from build123d import *

# Parameters (mm, degrees)
F1_DEPTH  = 1000
F2_T      = -3
F3_W      = 300
F3_H      = 3
F4_DEPTH  = 300
F6_DEPTH  = 5
F8_DEPTH  = 5
F9_W      = 100
F9_H      = 1500
F10_DEPTH = 100
F12_DEPTH = 800.001
F13_W     = 100
F13_H     = 1500
F14_DEPTH = 100
F16_DEPTH = 1100.001
F17_W     = 290
F17_H     = 3
F18_DEPTH = 300
F20_DEPTH = 5
F22_DEPTH = 5
F24_DEPTH = 100
F26_DEPTH = 100
F28_DEPTH = 744.22
F29_W     = 284.3456985965
F29_H     = 700
F30_DEPTH = 25.4


with BuildPart() as f1:
    # F0 (on Right) → F1 (new body)
    with BuildSketch(Plane.YZ):
        with BuildLine():
            Line((250, 100), (250, 600))
            Line((250, 600), (-250, 600))
            Line((-250, 600), (-250, 100))
            ThreePointArc((-250, 100), (-220.7106781187, 29.2893218813), (-150, 0))
            Line((-150, 0), (150, 0))
            ThreePointArc((150, 0), (220.7106781187, 29.2893218813), (250, 100))
        make_face()
    extrude(amount=F1_DEPTH)

    # F2
    f2_openings = [f1.faces().sort_by_distance(p)[0] for p in [
        (500, 0, 600),
    ]]
    offset(amount=F2_T, openings=f2_openings)

    # F3 (on face) → F4 (join)
    with BuildSketch(Plane(origin=(0, 0, 0), x_dir=(0, -1, 0), z_dir=(-1, 0, 0))):
        with Locations((0, 101.5)):
            Rectangle(F3_W, F3_H)
    extrude(amount=F4_DEPTH)

    # F5 (on face) → F6 (join)
    with BuildSketch(Plane.XZ.offset(150)):
        Polygon((0, 100), (-300, 100), (-300, 80), (0, 60), align=None)
    extrude(amount=-F6_DEPTH)

    # F7 (on face) → F8 (join)
    with BuildSketch(Plane(origin=(0, 150, 0), x_dir=(-1, 0, 0), z_dir=(0, 1, 0))):
        Polygon((300, 100), (0, 100), (0, 60), (300, 80), align=None)
    extrude(amount=-F8_DEPTH)

    # F9 (on face) → F10 (join)
    with BuildSketch(Plane.XZ.offset(250)):
        with Locations((250, -250)):
            Rectangle(F9_W, F9_H)
        with Locations((750, -250)):
            Rectangle(F9_W, F9_H)
    extrude(amount=F10_DEPTH)

    # F11 (on face) → F12 (cut, through all)
    with BuildSketch(Plane(origin=(200, 0, 0), x_dir=(0, -1, 0), z_dir=(-1, 0, 0))):
        Polygon((350, 500), (250, 500), (350, 400), align=None)
    extrude(amount=-F12_DEPTH, mode=Mode.SUBTRACT)

    # F13 (on face) → F14 (join)
    with BuildSketch(Plane(origin=(0, 250, 0), x_dir=(-1, 0, 0), z_dir=(0, 1, 0))):
        with Locations((-750, -250)):
            Rectangle(F13_W, F13_H)
        with Locations((-250, -250)):
            Rectangle(F13_W, F13_H)
    extrude(amount=F14_DEPTH)

    # F15 (on face) → F16 (cut, through all)
    with BuildSketch(Plane.YZ.offset(800)):
        Polygon((350, 500), (250, 500), (350, 400), align=None)
    extrude(amount=-F16_DEPTH, mode=Mode.SUBTRACT)

    # F17 (on face) → F18 (join)
    with BuildSketch(Plane.YZ.offset(1000)):
        with Locations((0, 101.5)):
            Rectangle(F17_W, F17_H)
    extrude(amount=F18_DEPTH)

    # F19 (on face) → F20 (join)
    with BuildSketch(Plane.XZ.offset(145)):
        Polygon((1300, 100), (1000, 100), (1000, 60), (1300, 80), align=None)
    extrude(amount=-F20_DEPTH)

    # F21 (on face) → F22 (join)
    with BuildSketch(Plane(origin=(0, 145, 0), x_dir=(-1, 0, 0), z_dir=(0, 1, 0))):
        Polygon((-1000, 100), (-1300, 100), (-1300, 80), (-1000, 60.6447160244), align=None)
    extrude(amount=-F22_DEPTH)

    # F23 (on face) → F24 (join, through all)
    with BuildSketch(Plane.XZ.offset(350)):
        Polygon((800, -758.5786437627), (800, -900), (1084.3456985965, -615.6543014035), (1013.6350204779, -544.9436232848), align=None)
    extrude(amount=-F24_DEPTH)

    # F25 (on face) → F26 (join)
    with BuildSketch(Plane(origin=(0, 350, 0), x_dir=(-1, 0, 0), z_dir=(0, 1, 0))):
        Polygon((-1084.3456985965, -615.6543014035), (-800, -900), (-800, -758.5786437627), (-1013.6350204779, -544.9436232848), align=None)
    extrude(amount=-F26_DEPTH)

    # F27 (on face) → F28 (cut)
    with BuildSketch(Plane.XZ.offset(350)):
        Polygon((942.9243423592, -615.6543014035), (1084.3456985965, -615.6543014035), (1013.6350204779, -544.9436232848), align=None)
    extrude(amount=-F28_DEPTH, mode=Mode.SUBTRACT)

    # F29 (on face) → F30 (join)
    with BuildSketch(Plane.XY.offset(-615.6543014035)):
        with Locations((942.1728492983, 0)):
            Rectangle(F29_W, F29_H)
    extrude(amount=F30_DEPTH)


solid = f1.part
Part model, mm, in its own coordinate system. A direction names the side the tool comes from. Give positions to 0.01 mm unless a question says otherwise; leave off trailing zeros. Loops run counter-clockwise (first coordinate to the right, second up) from the corner with the lowest first, then second, coordinate; pieces in that order, holes last. Notation, with made-up numbers: (58.25, 42) -> (65.25, 42) arc R19 cw to (65.25, 58) -> close; hole circle Ø7 at (69, 37.5). An arc over 180 degrees is marked (long way). Write each question's results on one line, items separated by ' | '. Start each with the question number.
Q1. Band-saw the part on B-B on z = -424.5. List the corners of the cut face in (x, y), plus the area to 3 significant figures.
Q2. Band-saw the part on A-A on y = -283.5. List the corners of the cut face in (x, z).
Q3. Pull direction X, two halves, no side cores. Call faces 4 (the face through (1148, -140, 85)), 5 (the face through (800, -299, -951)), 6 (the face through (300, -299, -260)): +X half, -X half, draft (parallel to the pull), parting line (faces both ways), or undercut.
Q4. Band-saw the part on C-C on y = -29. List the corners of the cut face in (x, z), plus the area to 3 significant figures.
Q5. Band-saw the part on D-D on x = 594. List the corners of the cut face in (y, z), plus the area to 3 significant figures.
Q6. Pin check, flat tips, straight feed: P1, Ø4, axis at x = 417.5, y = -217, coming from the +Z side; P2, Ø7.5, axis at y = -31, z = -607, coming from the +X side; P3, Ø8, axis at y = -25, z = 153, coming from the +X side. Stop position of each tip, or through.
Q7. Which spindle directions (+Z, -Z, +X, -X, +Y, -Y) get a long thin tool onto all of the face, cutting with end or side? Do faces 1 (the face through (-148, 145, 85)), 2 (the face through (493, -2, 0)), 3 (the face through (800, 299, -53)). Say none if no direction does.
Q8. Wall check: L1, parallel to Z at x = 905, y = -89.5; L2, parallel to Y at x = 901, z = 310.5; L3, parallel to X at y = -278, z = -756. Give the ranges that are in metal, low to high.
Results are:
1) outline: (200, -350) -> (300, -350) -> (300, -250) -> (200, -250) -> close; (200, 250) -> (300, 250) -> (300, 350) -> (200, 350) -> close; (700, -350) -> (800, -350) -> (800, -250) -> (700, -250) -> close; (700, 250) -> (800, 250) -> (800, 350) -> (700, 350) -> close | area: 40,000 mm²
2) outline: (200, -1000) -> (300, -1000) -> (300, 466.5) -> (200, 466.5) -> close; (700, -1000) -> (800, -1000) -> (800, -900) -> (1084.35, -615.65) -> (1084.35, -590.25) -> (800, -590.25) -> (800, 466.5) -> (700, 466.5) -> close; hole (800, -758.58) -> (942.92, -615.65) -> (800, -615.65) -> close
3) face 4: draft | face 5: +X half | face 6: undercut
4) outline: (-300, 100) -> (0, 100) -> (0, 0) -> (1000, 0) -> (1000, 100) -> (1300, 100) -> (1300, 103) -> (1000, 103) -> (1000, 600) -> (997, 600) -> (997, 3) -> (3, 3) -> (3, 600) -> (0, 600) -> (0, 103) -> (-300, 103) -> close; (800, -615.65) -> (1084.35, -615.65) -> (1084.35, -590.25) -> (800, -590.25) -> close | area: 15,600 mm²
5) outline: (-250, 100) arc R100 ccw to (-150, 0) -> (150, 0) arc R100 ccw to (250, 100) -> (250, 600) -> (247, 600) -> (247, 100) arc R97 cw to (150, 3) -> (-150, 3) arc R97 cw to (-247, 100) -> (-247, 600) -> (-250, 600) -> close | area: 4,830 mm²
6) P1: stops at z = 31.82 | P2: stops at x = 1084.35 | P3: stops at x = 1000
7) face 1: -Z, -X | face 2: +X, -X | face 3: +Z, +X, +Y
8) L1: z = -615.65 to -590.25, 0 to 3 | L2: y = -250 to -247, 247 to 250 | L3: x = 200 to 300, 700 to 800, 802.58 to 944
